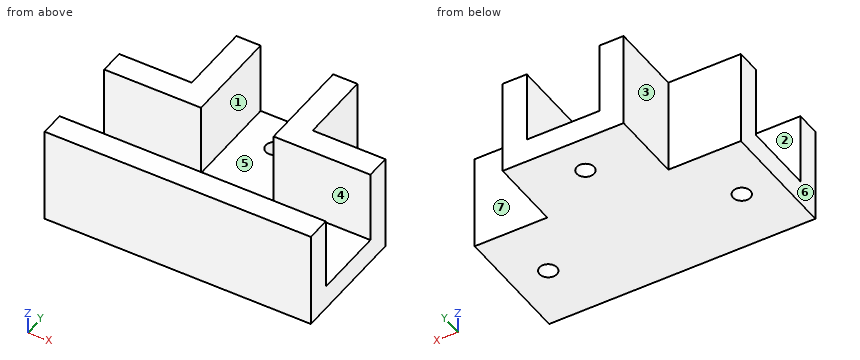
```python
from build123d import *

# Parameters (mm, degrees)
BOSS_EXTRUDE1_DEPTH = 5
BOSS_EXTRUDE2_DEPTH = 20
SKETCH4_W           = 55
SKETCH4_H           = 5
BOSS_EXTRUDE3_DEPTH = 20
SKETCH6_R           = 1.8
CUT_EXTRUDE3_DEPTH  = 6


with BuildPart() as part:
    # Sketch1 → Boss-Extrude1 (new body)
    with BuildSketch(Plane.XY):
        Polygon((14.31372549, -4.264705882), (34.31372549, -4.264705882), (34.31372549, -19.264705882), (-20.68627451, -19.264705882), (-20.68627451, -4.264705882), (-0.68627451, -4.264705882), (-0.68627451, 15.735294118), (14.31372549, 15.735294118), align=None)
    extrude(amount=BOSS_EXTRUDE1_DEPTH)

    # Sketch2 → Boss-Extrude2 (add)
    with BuildSketch(Plane(origin=(0, 0, 0), x_dir=(-1, 0, 0), z_dir=(0, 0, -1))):
        Polygon((0.68627451, 15.735294118), (5.68627451, 15.735294118), (5.68627451, 0.735294118), (6.079970528, 0.735294118), (20.68627451, 0.735294118), (20.68627451, -4.264705882), (0.68627451, -4.264705882), align=None)
    boss_extrude2 = extrude(amount=-BOSS_EXTRUDE2_DEPTH)

    # Sketch4 → Boss-Extrude3 (add)
    with BuildSketch(Plane(origin=(0, 0, 0), x_dir=(-1, 0, 0), z_dir=(0, 0, -1))):
        with Locations((-6.81372549, -21.764705882)):
            Rectangle(SKETCH4_W, SKETCH4_H)
    extrude(amount=-BOSS_EXTRUDE3_DEPTH)

    # Mirror1: Boss-Extrude2 across plane
    add(boss_extrude2.mirror(Plane.ZY.offset(-6.81372549)))

    # Sketch6 → Cut-Extrude3 (cut, through all)
    with BuildSketch(Plane.XY.offset(5)):
        with Locations((6.81372549, 8.235294118)):
            Circle(SKETCH6_R)
        with Locations((-13.18627451, -11.764705882)):
            Circle(SKETCH6_R)
        with Locations((26.81372549, -11.764705882)):
            Circle(SKETCH6_R)
    extrude(amount=-CUT_EXTRUDE3_DEPTH, mode=Mode.SUBTRACT)


solid = part.part
```
Source: CAD feature listing. Evaluate the final solid. Frame: model axes, mm. Face numbers are marked on the shaded views. A direction names the side the tool comes from. Coordinates: 2 decimals unless noted, no trailing zeros. Write each loop counter-clockwise with the first axis right and the second up, starting at its lowest first coordinate (ties: lowest second). Pieces come first, ordered by that corner, then holes. Notation, with made-up numbers: (-5.75, 6) - (40.25, 6) arc R20 ccw to (40.25, 30) - close; hole circle Ø8 at (38.5, 68.5). An arc over 180 degrees is marked (long way). Answer as a JSON object with one key per item and string values.
Q1. Section query C-C, the plane y = -11. Output: boundary loops of the cut face in (x, z), plus the area to 3 significant figures.
Ans:
{"outline": "(-20.69, 0) - (-14.82, 0) - (-14.82, 5) - (-20.69, 5) - close; (-11.56, 0) - (25.18, 0) - (25.18, 5) - (-11.56, 5) - close; (28.44, 0) - (34.31, 0) - (34.31, 5) - (28.44, 5) - close", "area": "242 mm2"}
Q2. Draft query along Y for the marked faces 4, 5, 6 and 7. Return one class per face: released by +Y, released by -Y, zero draft, split by the parting line, or undercut.
Ans:
{"face 4": "undercut", "face 5": "undercut", "face 6": "zero draft", "face 7": "released by +Y"}
Q3. Section query D-D, the plane z = 2.5. Output: boundary loops of the cut face in (x, y), plus the area to 3 significant figures.
Ans:
{"outline": "(-20.69, -24.26) - (34.31, -24.26) - (34.31, 0.74) - (19.31, 0.74) - (19.31, 15.74) - (-5.69, 15.74) - (-5.69, 0.74) - (-20.69, 0.74) - close; hole circle Ø3.6 at (-13.19, -11.76); hole circle Ø3.6 at (6.81, 8.24); hole circle Ø3.6 at (26.81, -11.76)", "area": "1,720 mm2"}
Q4. Section query A-A, the plane z = 13.5. Output: boundary loops of the cut face in (x, y), plus the area to 3 significant figures.
Ans:
{"outline": "(-20.69, -24.26) - (34.31, -24.26) - (34.31, -19.26) - (-20.69, -19.26) - close; (-20.69, -4.26) - (-0.69, -4.26) - (-0.69, 15.74) - (-5.69, 15.74) - (-5.69, 0.74) - (-20.69, 0.74) - close; (14.31, -4.26) - (34.31, -4.26) - (34.31, 0.74) - (19.31, 0.74) - (19.31, 15.74) - (14.31, 15.74) - close", "area": "625 mm2"}
Q5. First-contact query: pin 1 Ø4.5 at (x, z) = (-17, 6.5) entering from +Y; pin 2 Ø12 at (y, z) = (10, 10.5) entering from +X; pin 3 Ø7.5 at (y, z) = (6.5, 12.5) entering from -X; pin 4 Ø7.5 at (y, z) = (3.5, 15.5) entering from -X. Flat tips, straight axial feed; report the tip coordinate or a pass-through.
Ans:
{"pin 1": "stops at y = 0.74", "pin 2": "stops at x = 19.31", "pin 3": "stops at x = -5.69", "pin 4": "stops at x = -20.69"}
Q6. Material intervals for line 1 (X direction, y = 4, z = 5.25); line 2 (X direction, y = -2, z = 8.5); line 3 (Y direction, x = 27, z = 10.5), sorted ascending. Write a range as [from, to].
Ans:
{"line 1": "x = [-5.69, -0.69], [14.31, 19.31]", "line 2": "x = [-20.69, -0.69], [14.31, 34.31]", "line 3": "y = [-24.26, -19.26], [-4.26, 0.74]"}
Q7. Set-up query: the marked faces 1, 2 and 3. Return all of +Z, -Z, +X, -X, +Y, -Y with unobstructed straight access to the full face (end or side cutting, diameter ignored); none if empty.
Ans:
{"face 1": "+Z, +Y", "face 2": "+Z, +X, -X", "face 3": "+Z, -Z, -X, +Y"}
Q8. Section query B-B, the plane x = 23.5. Output: boundary loops of the cut face in (y, z).
Ans:
{"outline": "(-24.26, 0) - (0.74, 0) - (0.74, 20) - (-4.26, 20) - (-4.26, 5) - (-19.26, 5) - (-19.26, 20) - (-24.26, 20) - close"}
